Drawing for the job (mm, zero at the part's lowest x, y, z). Coordinates: 2 decimals unless noted, no trailing zeros. Write each loop counter-clockwise with the first axis right and the second up, starting at its lowest first coordinate (ties: lowest second). Pieces come first, ordered by that corner, then holes. Notation, with made-up numbers: M 87.25,67.5 L 102.25,67.5 A28 ccw 102.25,88.5 Z; hole C 39.25,-5 d6. An arc over 180 degrees is marked long. Put each result on its own line as item: value. Start each with the question number.
Q1. Cut at A-A (z = 5). Write the cut outline in (x, y) (1 decimal).
Q2. Cut at D-D (y = 8). Write the cut outline in (x, z) (1 decimal).
Q3. Drill centre lines: line 1 along Z through (x, y) = (58.5, 4) (1 decimal); line 2 along Y through (x, z) = (60.5, 5.25); line 3 along X through (y, z) = (80.5, 12) (1 decimal). Where is each one in solid material? Low to high.
Q4. Cut at B-B (x = 47). Write the cut outline in (y, z) (1 decimal).
Q5. Drop flat-ended pins along their axis: pin 1 (3 mm diameter, centred on y = 15, z = 5, fed in from +X); pin 2 (1.5 mm diameter, centred on y = 10.5, z = 11, fed in from -X) (1 decimal); pin 3 (7 mm diameter, centred on x = 6, z = 2.5, fed in from -Y); pin 4 (1.3 mm diameter, centred on x = 50.5, y = 1, fed in from +Z). Give the stop position or say it passes through.
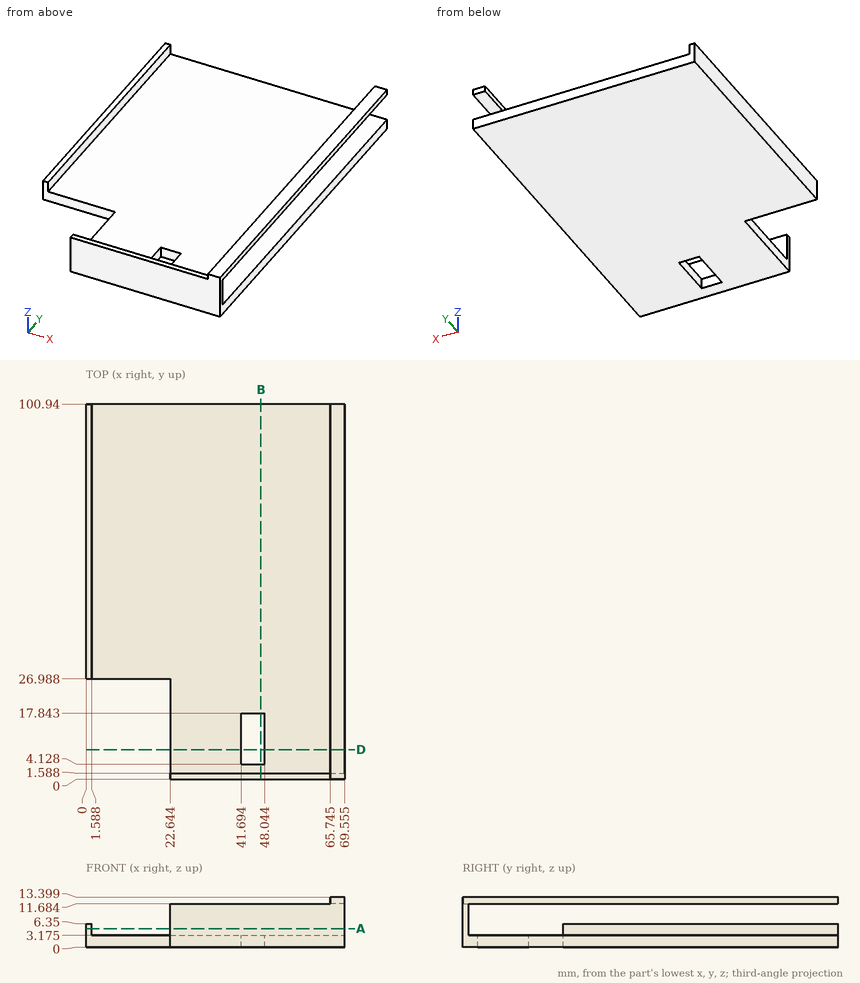
Computed values:
1. outline: M 0,27 L 1.6,27 L 1.6,100.9 L 0,100.9 Z; M 22.6,0 L 69.6,0 L 69.6,1.6 L 22.6,1.6 Z
2. outline: M 22.6,0 L 41.7,0 L 41.7,3.2 L 22.6,3.2 Z; M 48,0 L 69.6,0 L 69.6,3.2 L 48,3.2 Z; M 65.7,11.7 L 69.6,11.7 L 69.6,13.4 L 65.7,13.4 Z
3. line 1: 0 to 3.2
3. line 2: 0 to 1.59
3. line 3: 65.7 to 69.6
4. outline: M 0,0 L 4.1,0 L 4.1,3.2 L 1.6,3.2 L 1.6,11.7 L 0,11.7 Z; M 17.8,0 L 100.9,0 L 100.9,3.2 L 17.8,3.2 Z
5. pin 1: through
5. pin 2: x = 65.7
5. pin 3: y = 26.99
5. pin 4: z = 11.68
